Here's how the part is built. I have some questions about the finished solid (model axes, mm). A direction names the side the tool comes from. Coordinates: 2 decimals unless noted, no trailing zeros. Write each loop counter-clockwise with the first axis right and the second up, starting at its lowest first coordinate (ties: lowest second). Pieces come first, ordered by that corner, then holes. Notation, with made-up numbers: (34, -5) - (62, -5) arc R28 cw to (62, 28) - close; hole circle Ø4 at (74.5, -15.5). An arc over 180 degrees is marked (long way). Answer in a Markdown table with one row per item. Add a question column.
Item 1: Imagine slicing it at D-D (y = -508). Please give me the cut outline in (x, z).
Item 2: We'd pull the mould along Z, two halves only. Please class faces 1 (the face through (-50, -330.2, 48)), 2 (the face through (-2, 269, -63.724)), 3 (the face through (5.506, 34.707, -24.796)): +Z half, -Z half, draft (parallel to the pull), parting line (faces both ways), or undercut.
Item 3: Imagine slicing it at C-C (x = 0). Please give me the cut outline in (y, z), plus the area to 3 significant figures.
Item 4: If I drill on probe 1 along Z at (x, y) = (-2, 189.5); probe 2 along Z at (x, y) = (0, -273); probe 3 along X at (y, z) = (-407.5, 10), over which ranges is the centre line in solid material (lowest first)? Write a range as from..to.
Item 5: Imagine slicing it at A-A (z = 0). Please give me the cut outline in (x, y), plus the area to 3 significant figures.
Item 6: Which directions (+Z, -Z, +X, -X, +Y, -Y) give clear straight access to the entire face, cutting with the end or side of a thin tool? Please do faces 4 (the face through (53.719, -455.6, 16.917)), 5 (the face through (86.914, 160, -2)).
Item 7: I'm going to push flat-ended pins straight in: pin 1 (2 mm diameter, centred on y = -330.5, z = 12.5, fed in from +X); pin 2 (8 mm diameter, centred on y = -433, z = -55, fed in from +X); pin 3 (1 mm diameter, centred on x = 31.5, y = 159, fed in from +Z). Where does each tip first touch, or does it pass through?
Item 8: Imagine slicing it at B-B (y = -154.5). Please give me the cut outline in (x, z), plus the area to 3 significant figures.
from build123d import *

# Parameters (mm, degrees)
F0_R          = 76.8686111214
F1_DEPTH      = 254
F2_W          = 175.2306818962
F2_H          = 125.6063729525
F3_DEPTH      = 890.52474
F4_R          = 58.9166672022
F3_FACE1_W    = 175.2306818962
F3_FACE1_H    = 125.6063729525
F5_DEPTH      = 76.2
F6_R          = 56.3193405809
F7_DEPTH      = 254
F7_DEPTH_BACK = 25.4
F8_R          = 12.7
F9_R          = 12.7
F11_D         = 50.8
F12_R         = 5.08


with BuildPart() as f1:
    # F0 (on Front) → F1 (new body)
    with BuildSketch(Plane.XZ):
        Circle(F0_R)
    extrude(amount=F1_DEPTH)

    # F2 (on face) → F3 (join)
    with BuildSketch(Plane.XZ.offset(254)):
        with Locations((-0.7015764713, -0.9209215641)):
            Rectangle(F2_W, F2_H)
        with BuildLine():
            Line((86.9137644768, 61.8822649121), (45.6000950117, 61.8822649121))
            ThreePointArc((45.6000950117, 61.8822649121), (68.6075773741, 34.6667521206), (76.8686111214, 0))
            ThreePointArc((76.8686111214, 0), (67.8721550854, -36.0853701628), (42.9886197754, -63.7241080403))
            Line((42.9886197754, -63.7241080403), (86.9137644768, -63.7241080403))
            Line((86.9137644768, -63.7241080403), (86.9137644768, 61.8822649121))
        make_face()
    extrude(amount=-F3_DEPTH)

    # F4 (on face) + F3_face (on face) + F3_face1 (on face) → F5 (join)
    with BuildSketch(Plane.XZ.offset(254)):
        Circle(F4_R)
    with BuildSketch(Plane(origin=(-0.6513319222, -254, -0.4226097365), x_dir=(1, 0, 0), z_dir=(0, -1, 0))):
        with BuildLine():
            Line((43.6399516976, -63.3014983039), (87.565096399, -63.3014983039))
            Line((87.565096399, -63.3014983039), (87.565096399, 62.3048746486))
            Line((87.565096399, 62.3048746486), (46.2514269339, 62.3048746486))
            ThreePointArc((46.2514269339, 62.3048746486), (0.6513319222, 77.2912208578), (-44.9487630895, 62.3048746486))
            Line((-44.9487630895, 62.3048746486), (-87.6655854972, 62.3048746486))
            Line((-87.6655854972, 62.3048746486), (-87.6655854972, -63.3014983039))
            Line((-87.6655854972, -63.3014983039), (-42.3372878532, -63.3014983039))
            ThreePointArc((-42.3372878532, -63.3014983039), (0.6513319222, -76.4460013849), (43.6399516976, -63.3014983039))
        make_face()
    with BuildSketch(Plane(origin=(-0.7015764713, 636.52474, -0.9209215641), x_dir=(1, 0, 0), z_dir=(0, 1, 0))):
        Rectangle(F3_FACE1_W, F3_FACE1_H)
    extrude(amount=F5_DEPTH, dir=(0, -1, 0))

    # F6 (on face) → F7 (join, two sides)
    with BuildSketch(Plane.XZ.offset(330.2)) as f7_sk:
        Circle(F6_R)
    extrude(amount=F7_DEPTH)
    extrude(f7_sk.sketch, amount=-F7_DEPTH_BACK)

    # F8
    f8_edges = [f1.edges().sort_by_distance(p)[0] for p in [
        (-56.319341, -330.2, 0),
    ]]
    fillet(f8_edges, radius=F8_R)

    # F9
    f9_edges = [f1.edges().sort_by_distance(p)[0] for p in [
        (-56.319341, -584.2, 0),
    ]]
    fillet(f9_edges, radius=F9_R)

    # F11 (through all)
    with Locations(Plane.XZ.offset(584.2)):
        with Locations((0, 0)):
            Hole(F11_D / 2)

    # F12
    f12_edges = [f1.edges().sort_by_distance(p)[0] for p in [
        (86.913764, 153.16237, 61.882265),
        (-88.316917, 153.16237, 61.882265),
        (86.913764, 153.16237, -63.724108),
        (86.913764, -330.2, -0.920922),
        (-88.316917, -330.2, -0.920922),
        (86.913764, 636.52474, -0.920922),
        (-0.701576, 636.52474, 61.882265),
        (-88.316917, 153.16237, -63.724108),
        (-65.652769, -330.2, -63.724108),
        (64.951192, -330.2, -63.724108),
        (0, -330.2, 76.868611),
        (0, -330.2, -76.868611),
        (66.25693, -330.2, 61.882265),
        (-88.316917, 636.52474, -0.920922),
    ]]
    fillet(f12_edges, radius=F12_R)


solid = f1.part
Here are the results:
| question | item | result |
|---|---|---|
| 1 | outline | circle Ø112.64 at (0, 0); hole circle Ø50.8 at (0, 0) |
| 2 | face 1 | draft |
| 2 | face 2 | -Z half |
| 2 | face 3 | undercut |
| 3 | outline | (-584.2, -43.62) arc R12.7 ccw to (-571.5, -56.32) - (-342.9, -56.32) arc R12.7 cw to (-330.2, -69.02) - (-330.2, -71.79) arc R5.08 ccw to (-325.12, -76.87) - (0, -76.87) - (0, -63.72) - (636.52, -63.72) - (636.52, -25.4) - (-584.2, -25.4) - close; (-584.2, 25.4) - (636.52, 25.4) - (636.52, 56.8) arc R5.08 ccw to (631.44, 61.88) - (0, 61.88) - (0, 76.87) - (-325.12, 76.87) arc R5.08 ccw to (-330.2, 71.79) - (-330.2, 69.02) arc R12.7 cw to (-342.9, 56.32) - (-571.5, 56.32) arc R12.7 ccw to (-584.2, 43.62) - close |
| 3 | area | 97,300 mm2 |
| 4 | probe 1 | z = -63.72..-25.32, 25.32..61.88 |
| 4 | probe 2 | z = -76.87..-25.4, 25.4..76.87 |
| 4 | probe 3 | x = -55.42..-23.35, 23.35..55.42 |
| 5 | outline | (-88.32, -325.12) arc R5.08 ccw to (-83.24, -330.2) - (-69.02, -330.2) arc R12.7 cw to (-56.32, -342.9) - (-56.32, -571.5) arc R12.7 ccw to (-43.62, -584.2) - (-25.4, -584.2) - (-25.4, 636.52) - (-83.24, 636.52) arc R5.08 ccw to (-88.32, 631.44) - close; (25.4, -584.2) - (43.62, -584.2) arc R12.7 ccw to (56.32, -571.5) - (56.32, -342.9) arc R12.7 cw to (69.02, -330.2) - (81.83, -330.2) arc R5.08 ccw to (86.91, -325.12) - (86.91, 631.44) arc R5.08 ccw to (81.83, 636.52) - (25.4, 636.52) - close |
| 5 | area | 136,000 mm2 |
| 6 | face 4 | -Y |
| 6 | face 5 | +Z, -Z, +X, +Y, -Y |
| 7 | pin 1 | stops at x = 84.41 |
| 7 | pin 2 | stops at x = 23.89 |
| 7 | pin 3 | stops at z = 61.88 |
| 8 | outline | (-88.32, -58.64) arc R5.08 ccw to (-83.24, -63.72) - (-42.99, -63.72) arc R76.87 ccw to (42.99, -63.72) - (81.83, -63.72) arc R5.08 ccw to (86.91, -58.64) - (86.91, 56.8) arc R5.08 ccw to (81.83, 61.88) - (45.6, 61.88) arc R76.87 ccw to (-45.6, 61.88) - (-83.24, 61.88) arc R5.08 ccw to (-88.32, 56.8) - close; hole circle Ø50.8 at (0, 0) |
| 8 | area | 21,700 mm2 |
